from build123d import *

# Parameters (mm, degrees)
F1_DEPTH = 25.4
F2_T     = -22.225
F4_D     = 12.7


with BuildPart() as f1:
    # F0 (on Top) → F1 (new body)
    with BuildSketch(Plane.XY):
        Polygon((-147.42167, 108.847304), (-178.948584, 39.475165), (-179.533662, -36.722589), (-149.075739, -106.570674), (-92.841266, -157.991721), (-20.553695, -182.094564), (55.287797, -174.711602), (121.569526, -137.119418), (166.83078, -75.81804), (183.245477, -1.407035), (167.975366, 73.24726), (123.660788, 135.236438), (57.964136, 173.842007), (-17.755041, 182.388714), (-90.40421, 159.398755), align=None)
    extrude(amount=F1_DEPTH)

    # F2
    f2_openings = [f1.faces().sort_by_distance(p)[0] for p in [
        (0, 0, 25.4),
    ]]
    offset(amount=F2_T, openings=f2_openings)

    # F4 (through all)
    with Locations(Plane(origin=(88.428662, -155.91551, 0), x_dir=(0.869839, 0.493336, 0), z_dir=(0.493336, -0.869839, 0))):
        with Locations((0, 15.245483)):
            Hole(F4_D / 2)


solid = f1.part
The model under review builds one solid part; all positions refer to its coordinate system, in mm. A direction names the side the tool comes from. Coordinates: 2 decimals unless noted, no trailing zeros. Write each loop counter-clockwise with the first axis right and the second up, starting at its lowest first coordinate (ties: lowest second). Pieces come first, ordered by that corner, then holes. Notation, with made-up numbers: (-13, 19.25) -> (11, 19.25) arc R18 cw to (11, 33.25) -> close; hole circle Ø4 at (-13, 6). An arc over 180 degrees is marked (long way). Answer in a Markdown table with one row per item.
1. We need section B-B, the plane x = -101.5. State the section outline as (y, z) points (3 decimals).
Answers below:
| item | result |
|---|---|
| outline | (-150.074, 0) -> (149.561, 0) -> (149.561, 25.4) -> (119.859, 25.4) -> (119.859, 22.225) -> (-119.958, 22.225) -> (-119.958, 25.4) -> (-150.074, 25.4) -> close |
2. Wall thickness on probe 1 along Z at (x, y) = (-43, 144) (3 decimals); probe 2 along X at (y, z) = (10.5, 12.5); probe 3 along Y at (x, z) = (63.5, 23.75): over which ranges is each line inside the solid? List them lowest first. Write a range as [from, to].
Answers below:
| item | result |
|---|---|
| probe 1 | z = [0, 22.225] |
| probe 2 | x = [-179.17, -12.54], [0.63, 180.81] |
| probe 3 | y = [-170.05, -144.5], [144.81, 170.59] |
3. Draft analysis for pull direction Y (two halves, no side actions). For faces 1 (the flat face through (153.93, 31.01, 23.79)), 2 (the flat face through (16.836, -178.455, 12.522)), 3 (the flat face through (146.128, 103.808, 12.522)), 4 (the flat face through (-120, -107, 25.4)), state which applies: +Y half, -Y half, draft (parallel to the pull), parting line (faces both ways), or undercut.
Answers below:
| item | result |
|---|---|
| face 1 | undercut |
| face 2 | -Y half |
| face 3 | +Y half |
| face 4 | draft |
4. We need section A-A, the plane z = 4. State the section outline as (x, y) points.
Answers below:
| item | result |
|---|---|
| outline | (-179.53, -36.72) -> (-149.08, -106.57) -> (-92.84, -157.99) -> (-20.55, -182.09) -> (55.29, -174.71) -> (121.57, -137.12) -> (166.83, -75.82) -> (183.25, -1.41) -> (167.98, 73.25) -> (123.66, 135.24) -> (57.96, 173.84) -> (-17.76, 182.39) -> (-90.4, 159.4) -> (-147.42, 108.85) -> (-178.95, 39.48) -> close |
5. Clearance check with flat-ended pins moving along their axes: pin 1 Ø1 at (y, z) = (1, 7.5) entering from -X; pin 2 Ø8 at (y, z) = (-51, 13) entering from -X; pin 3 Ø6 at (x, z) = (58.5, 20.5) entering from +Y. State where each tip first meets the part, or that it passes through.
Answers below:
| item | result |
|---|---|
| pin 1 | stops at x = -179.25 |
| pin 2 | stops at x = -175.05 |
| pin 3 | stops at y = 174.12 |
6. For faces 5 (the flat face through (128.01, 90.937, 23.79)), 6 (the flat face through (-1, 3, 0)), list the 3-axis set-ups (+Z, -Z, +X, -X, +Y, -Y) from which the entire face can be reached by the end or side of a thin tool; tool diameter is ignored.
Answers below:
| item | result |
|---|---|
| face 5 | +Z |
| face 6 | -Z, +X, -X, +Y, -Y |
